from build123d import *

# Parameters (mm, degrees)
F2_DEPTH = 750
F3_DEPTH = 100
F5_START = 100
F5_DEPTH = 200
F6_SIZE  = 2.54
F7_SIZE  = 2.54
F9_D     = 5


with BuildPart() as f2:
    # F0 (on Top) → F2 (new body)
    with BuildSketch(Plane.XY):
        with BuildLine():
            Line((-25.4, 0), (25.4, 0))
            ThreePointArc((25.4, 0), (0, 25.4), (-25.4, 0))
        make_face()
    extrude(amount=-F2_DEPTH)

    # F1 (on Top) → F3 (join)
    with BuildSketch(Plane.XY):
        with BuildLine():
            Line((-25.4, 0), (25.4, 0))
            ThreePointArc((25.4, 0), (25.2146859333, 3.0626154324), (24.6614477727, 6.0805422254))
            Line((24.6614477727, 6.0805422254), (11.4050507545, 6.0805422254))
            Line((11.4050507545, 6.0805422254), (14.879071159, 20.5857533611))
            ThreePointArc((14.879071159, 20.5857533611), (0, 25.4), (-14.879071159, 20.5857533611))
            Line((-14.879071159, 20.5857533611), (-11.4050507545, 6.0805422254))
            Line((-11.4050507545, 6.0805422254), (-24.6614477727, 6.0805422254))
            ThreePointArc((-24.6614477727, 6.0805422254), (-25.2146859333, 3.0626154324), (-25.4, 0))
        make_face()
    extrude(amount=F3_DEPTH)

    # F4 (on Top) → F5 (join)
    with BuildSketch(Plane.XY.offset(F5_START)):
        with BuildLine():
            Line((-25.4, 0), (25.4, 0))
            ThreePointArc((25.4, 0), (0, 25.4), (-25.4, 0))
        make_face()
    extrude(amount=F5_DEPTH)

    # F6
    f6_edges = [f2.edges().sort_by_distance(p)[0] for p in [
        (0, 25.4, -750),
    ]]
    chamfer(f6_edges, length=F6_SIZE)

    # F7
    f7_edges = [f2.edges().sort_by_distance(p)[0] for p in [
        (0, 25.4, 300),
    ]]
    chamfer(f7_edges, length=F7_SIZE)

    # F9 (through all)
    with Locations(Plane.XZ):
        with Locations((0, -50)):
            Hole(F9_D / 2)


solid = f2.part
The model under review builds one solid part; all positions refer to its coordinate system, in mm. Coordinates: 2 decimals unless noted, no trailing zeros. Loops run counter-clockwise (first coordinate to the right, second up) from the corner with the lowest first, then second, coordinate; pieces in that order, holes last. Notation, with made-up numbers: (-24, 77) -> (35, 77) arc R6 cw to (35, 86) -> close; hole circle Ø9 at (48.5, -25.5). An arc over 180 degrees is marked (long way). Use a Markdown table: item, result. Add a question column.
1. Clearance check with flat-ended pins moving along their axes: pin 1 Ø12 at (x, z) = (11, -108) entering from +Y; pin 2 Ø6.5 at (x, z) = (-21.5, 38.5) entering from +Y; pin 3 Ø14.5 at (x, z) = (17, 40) entering from +Y. State where each tip first meets the part, or that it passes through.
2. Add section A-A on z = -420. Write out the cut boundary in (x, y), plus the area to 3 significant figures.
3. To check wall thickness, follow line 1 (Z direction, x = -0.5, y = 20.75); line 2 (Z direction, x = 0, y = 19); line 3 (Y direction, x = -6, z = -684). State the ranges of each line that lie inside material, in increasing order.
Returned:
| question | item | result |
|---|---|---|
| 1 | pin 1 | stops at y = 24.9 |
| 1 | pin 2 | stops at y = 6.08 |
| 1 | pin 3 | stops at y = 23.45 |
| 2 | outline | (-25.4, 0) -> (25.4, 0) arc R25.4 ccw to start |
| 2 | area | 1,010 mm² |
| 3 | line 1 | z = -750 to -52.45, -47.55 to 300 |
| 3 | line 2 | z = -750 to -52.5, -47.5 to 300 |
| 3 | line 3 | y = 0 to 24.68 |
